from build123d import *

# Parameters (mm, degrees)
SKETCH1_R           = 15
BOSS_EXTRUDE1_DEPTH = 72
SKETCH3_R           = 15
SKETCH3_R_2         = 7.5
BOSS_EXTRUDE2_DEPTH = 17
BOSS_EXTRUDE3_START = -5
SKETCH4_R           = 22.5
SKETCH4_R_2         = 12.5
SKETCH4_R_3         = 2
BOSS_EXTRUDE3_DEPTH = 5
SKETCH6_R           = 6
SKETCH6_R_2         = 3
BOSS_EXTRUDE4_DEPTH = 35
CUT_EXTRUDE2_START  = -67
SKETCH9_R           = 7.5
CUT_EXTRUDE2_DEPTH  = 67
CUT_EXTRUDE3_START  = -5
SKETCH10_R          = 3
CUT_EXTRUDE3_DEPTH  = 5
FILLET1_R           = 10
FILLET2_R           = 2
BOSS_EXTRUDE5_START = -84
SKETCH12_R          = 7.5
BOSS_EXTRUDE5_DEPTH = 84


with BuildPart() as part:
    # Sketch1 → Boss-Extrude1 (new body)
    with BuildSketch(Plane.XY):
        Circle(SKETCH1_R)
    extrude(amount=BOSS_EXTRUDE1_DEPTH)

    # Sketch3 → Boss-Extrude2 (add)
    with BuildSketch(Plane.XY.offset(72)):
        Circle(SKETCH3_R)
        Circle(SKETCH3_R_2, mode=Mode.SUBTRACT)
    extrude(amount=BOSS_EXTRUDE2_DEPTH)

    # Sketch4 → Boss-Extrude3 (add)
    with BuildSketch(Plane.XY.offset(89).offset(BOSS_EXTRUDE3_START)):
        Circle(SKETCH4_R)
        Circle(SKETCH4_R_2, mode=Mode.SUBTRACT)
        with Locations((0, 18.75)):
            Circle(SKETCH4_R_3, mode=Mode.SUBTRACT)
        with Locations((16.237976321, 9.375)):
            Circle(SKETCH4_R_3, mode=Mode.SUBTRACT)
        with Locations((16.237976321, -9.375)):
            Circle(SKETCH4_R_3, mode=Mode.SUBTRACT)
        with Locations((0, -18.75)):
            Circle(SKETCH4_R_3, mode=Mode.SUBTRACT)
        with Locations((-16.237976321, -9.375)):
            Circle(SKETCH4_R_3, mode=Mode.SUBTRACT)
        with Locations((-16.237976321, 9.375)):
            Circle(SKETCH4_R_3, mode=Mode.SUBTRACT)
    extrude(amount=-BOSS_EXTRUDE3_DEPTH)

    # Sketch6 → Boss-Extrude4 (add)
    with BuildSketch(Plane(origin=(0, 0, 0), x_dir=(-1, 0, 0), z_dir=(0, 0, -1))):
        with Locations(Location((0, 0, 0), (0, 0, 180))):
            Circle(SKETCH6_R)
        Circle(SKETCH6_R_2, mode=Mode.SUBTRACT)
    extrude(amount=BOSS_EXTRUDE4_DEPTH)

    # Sketch9 → Cut-Extrude2 (cut)
    with BuildSketch(Plane.XY.offset(72).offset(CUT_EXTRUDE2_START)):
        Circle(SKETCH9_R)
    extrude(amount=CUT_EXTRUDE2_DEPTH, mode=Mode.SUBTRACT)

    # Sketch10 → Cut-Extrude3 (cut)
    with BuildSketch(Plane(origin=(0, 0, 0), x_dir=(-1, 0, 0), z_dir=(0, 0, -1)).offset(CUT_EXTRUDE3_START)):
        with Locations(Location((0, 0, 0), (0, 0, 180))):
            Circle(SKETCH10_R)
    extrude(amount=CUT_EXTRUDE3_DEPTH, mode=Mode.SUBTRACT)

    # Fillet1
    # the kernel refuses this fillet: 10 mm, written as the material it adds along each edge
    with BuildSketch(Plane(origin=(0, 0, 0), x_dir=(1, 0, 0), z_dir=(0, 1, 0))) as fillet1_piece_1:
        with BuildLine():
            CenterArc((16, 9.949874371), FILLET1_R, 180, 84.260829523)
            Line((6, 9.949874371), (5.8, 9.949874371))
            Line((5.8, 9.949874371), (5.8, 0))
            Line((5.8, 0), (6, -0.2))
            ThreePointArc((6, -0.2), (10.5, -0.2), (14.98, -0.198997487))
            Line((14.98, -0.198997487), (15, 0))
        make_face()
    revolve(axis=Axis((0, 0, 0), (0, 0, -1)))

    # Fillet2
    fillet2_edges = [part.edges().sort_by_distance(p)[0] for p in [
        (-15, 0, 0),
    ]]
    fillet(fillet2_edges, radius=FILLET2_R)

    # Sketch12 → Boss-Extrude5 (add)
    with BuildSketch(Plane.XY.offset(89).offset(BOSS_EXTRUDE5_START)):
        Circle(SKETCH12_R)
    extrude(amount=BOSS_EXTRUDE5_DEPTH)


solid = part.part
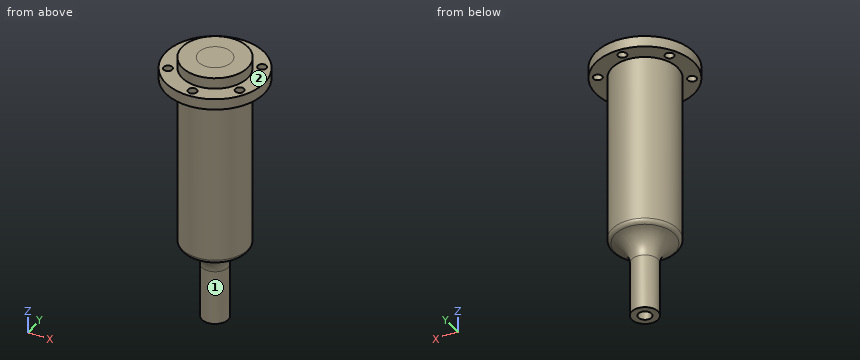
Geometry check sheet. Reference: the model listing, model coordinates, mm. Face numbers are marked on the shaded views. A direction names the side the tool comes from. Give positions to 0.01 mm unless a question says otherwise; leave off trailing zeros. Write each loop counter-clockwise with the first axis right and the second up, starting at its lowest first coordinate (ties: lowest second). Pieces come first, ordered by that corner, then holes.
1) Cross-section at C-C (z = 14). Record the boundary of the cut face in (x, y).
Values follow:
outline: circle Ø30 at (0, 0)
2) Set-up check for the marked faces 1 and 2: record each of +Z, -Z, +X, -X, +Y, -Y from which the full face is reachable in a straight line by a thin tool's end or side.
Values follow:
face 1: -Z
face 2: +Z
3) Cross-section at A-A (y = -18.75). Record the boundary of the cut face in (x, z).
Values follow:
outline: (-12.44, 79) - (-2, 79) - (-2, 84) - (-12.44, 84) - close; (2, 79) - (12.44, 79) - (12.44, 84) - (2, 84) - close
4) Thickness scan on line 1 (Z direction, x = 8, y = 14); line 2 (X direction, y = -0.5, z = 23); line 3 (X direction, y = -3.5, z = 31). Record the ranges inside material, lowest first.
Values follow:
line 1: z = 79 to 84
line 2: x = -14.99 to 14.99
line 3: x = -14.59 to 14.59
5) Go/stop test with flat-tipped pins: pin 1 Ø3.5 at (x, y) = (0, 18.75) entering from -Z; pin 2 Ø5 at (x, y) = (-16.24, -9.38) entering from -Z; pin 3 Ø12 at (x, z) = (0.5, 75.5) entering from +Y; pin 4 Ø5 at (x, y) = (16.24, 9.38) entering from +Z. Record where each tip stops, or that it passes through.
Values follow:
pin 1: passes through
pin 2: stops at z = 79
pin 3: stops at y = 22.5
pin 4: stops at z = 84
6) Cross-section at B-B (x = 0). Count the separate pieces of the cut face and the enclosed holes in it, plus the area to 3 significant figures.
Values follow:
separate pieces: 3
enclosed holes: 0
area: 2,930 mm2
